For this review, take the finished solid that the model builds, in its own axes (mm). A direction names the side the tool comes from. Round coordinates to 2 decimals unless told otherwise and drop trailing zeros. Write each loop counter-clockwise with the first axis right and the second up, starting at its lowest first coordinate (ties: lowest second). Pieces come first, ordered by that corner, then holes. Notation, with made-up numbers: M 44.5,-5.75 L 64.5,-5.75 A35 cw 64.5,31.25 Z; hole C 54.5,-25 d7. An arc over 180 degrees is marked long. Use one line per item in the form item = value. Start each with the question number.
Item 1: Add section B-B (z = 7.5). State the section outline as (x, y) points.
Item 2: Add section A-A (y = 0). State the section outline as (x, z) points.
Item 3: Add section D-D (z = 45.5). State the section outline as (x, y) points, and give its area (3 significant figures).
Item 4: For faces 1 (the flat face through (-88, -12.7, 13)), 2 (the cylindrical face through (-189.067, -5.86, 38.361)), list the 3-axis set-ups (+Z, -Z, +X, -X, +Y, -Y) from which the entire face can be reached by the end or side of a thin tool; tool diameter is ignored.
Item 5: For line 1 (Z direction, x = -3, y = -9.5); line 2 (X direction, y = 11, z = 39); line 3 (Y direction, x = -177, z = 41), list the stretches that pass through material, from the lowest coordinate up. Write a range as [from, to].
Item 6: Add section C-C (x = -62.5). State the section outline as (y, z) points, and give its area (3 significant figures).
Item 7: For P1, Ø12.5, axis at x = -107, y = 5, coming from the +Z side; P2, Ø1.5, axis at y = -0.5, z = 21, coming from the +X side; P3, Ø5, axis at y = -5.5, z = 29, coming from the -X side; P4, Ø4, axis at y = -4.5, z = 23.5, coming from the -X side, all flat-tipped, find the tip position at first contact; note any pin that passes through.
from build123d import *

# Parameters (mm, degrees)
BOSS_EXTRUDE1_DEPTH = 25.4
SKETCH2_R           = 12.7
BOSS_EXTRUDE2_DEPTH = 38.1


with BuildPart() as part:
    # Sketch1 → Boss-Extrude1 (new body)
    with BuildSketch(Plane.XY):
        with BuildLine():
            Line((0, -12.7), (-177.8, -12.7))
            ThreePointArc((-177.8, -12.7), (-190.5, 0), (-177.8, 12.7))
            Line((-177.8, 12.7), (0, 12.7))
            ThreePointArc((0, 12.7), (12.7, 0), (0, -12.7))
        make_face()
    extrude(amount=BOSS_EXTRUDE1_DEPTH)

    # Sketch2 → Boss-Extrude2 (add)
    with BuildSketch(Plane.XY.offset(25.4)):
        with Locations(Location((-177.8, 0, 0), (0, 0, 270))):
            Circle(SKETCH2_R)
    extrude(amount=BOSS_EXTRUDE2_DEPTH)


solid = part.part
Calculated:
q1.outline = M -177.8,-12.7 L 0,-12.7 A12.7 ccw 0,12.7 L -177.8,12.7 A12.7 ccw Z
q2.outline = M -190.5,0 L 12.7,0 L 12.7,25.4 L -165.1,25.4 L -165.1,63.5 L -190.5,63.5 Z
q3.outline = C -177.8,0 d25.4
q3.area = 507 mm^2
q4.face_1 = +Z, -Z, +X, -X, -Y
q4.face_2 = +Z
q5.line_1 = [0, 25.4]
q5.line_2 = [-184.15, -171.45]
q5.line_3 = [-12.67, 12.67]
q6.outline = M -12.7,0 L 12.7,0 L 12.7,25.4 L -12.7,25.4 Z
q6.area = 645 mm^2
q7.P1 = 25.4
q7.P2 = 12.7
q7.P3 = -190.14
q7.P4 = -190.25
